Source: CAD feature listing. Evaluate the final solid. Frame: model axes, mm. Face numbers are marked on the shaded views. Round coordinates to 2 decimals unless told otherwise and drop trailing zeros. Order: outer loops, then holes, each group sorted by start corner. A loop starts at its lowest first (then second) coordinate and runs counter-clockwise, first axis right, second up. Notation, with made-up numbers: (6, 38) -> (46, 38) arc R28 cw to (46, 62) -> close; hole circle Ø1 at (40, 88). An arc over 180 degrees is marked (long way). Write item = value, one per line. Start each with the question number.
(1) Cut plane C-C on z = 12. Return the cut outline in (x, y) (3 decimals), then the cut area to 3 significant figures.
(2) Ray query, line 1 (Y direction, x = 11.71, z = 0.6); line 2 (X direction, y = 2.75, z = 1); line 3 (Y direction, x = 11.71, z = 5.75). Return the intervals inside material, ascending.
(3) Contact query for a flat-ended pin moving along its axis: pin 1 Ø2 at (x, y) = (8.5, 1) entering from +Z. Output: stop coordinate, or through.
(4) Cut plane A-A on x = 27.29. Return the cut outline in (y, z).
(5) Cut plane B-B on z = 3. Return the cut outline in (x, y) (3 decimals), then the cut area to 3 significant figures.
(6) Draft query along Y for the marked faces 1, 2, 3 and 4. Return one class per face: released by +Y, released by -Y, zero draft, split by the parting line, or undercut.
(7) Cut plane D-D on y = 3. Give the number of separate pieces and of enclosed holes in the cut face, then the cut area to 3 significant figures.
from build123d import *

# Parameters (mm, degrees)
SKETCH1_W                = 39
SKETCH1_H                = 7.38
BOSS_EXTRUDE1_DEPTH      = 7.76
SKETCH2_R                = 2.4
CUT_EXTRUDE1_DEPTH       = 7.76
CUT_EXTRUDE2_OUTLINE_R   = 3.1
CUT_EXTRUDE2_OUTLINE_R_2 = 2.4
CUT_EXTRUDE2_DEPTH       = 0.8
CUT_EXTRUDE3_START       = 6.96
CUT_EXTRUDE3_OUTLINE_R   = 3.1
CUT_EXTRUDE3_OUTLINE_R_2 = 2.4
CUT_EXTRUDE3_DEPTH       = 0.8
LPATTERN3_COUNT          = 3
LPATTERN3_PITCH          = 7.79
LPATTERN6_COUNT          = 3
LPATTERN6_PITCH          = 7.79
FILLET1_R                = 3.69
FILLET2_R                = 3.69
FILLET3_R                = 3.69
FILLET4_R                = 3.69
SKETCH3_R                = 3.1
BOSS_EXTRUDE2_DEPTH      = 7.76
BOSS_EXTRUDE3_START      = -7.76
SKETCH4_R                = 3.1
BOSS_EXTRUDE3_DEPTH      = 7.76
SKETCH11_R               = 1.555
BOSS_EXTRUDE7_DEPTH      = 8
SKETCH12_R               = 1.555
BOSS_EXTRUDE8_DEPTH      = 8
SKETCH14_R               = 1.555
BOSS_EXTRUDE9_DEPTH      = 8


# Read off the part's stored shape, not the designer's step: Cut-Extrude2, Cut-Extrude3
with BuildPart() as part:
    # Sketch1 → Boss-Extrude1 (new body)
    with BuildSketch(Plane.XY):
        with Locations((19.5, 3.69)):
            Rectangle(SKETCH1_W, SKETCH1_H)
    extrude(amount=BOSS_EXTRUDE1_DEPTH)

    # Sketch2 → Cut-Extrude1 (cut)
    with BuildSketch(Plane.XY.offset(7.76)):
        with Locations((19.5, 3.69)):
            Circle(SKETCH2_R)
    cut_extrude1 = extrude(amount=-CUT_EXTRUDE1_DEPTH, mode=Mode.SUBTRACT)

    # Cut-Extrude2 outline → Cut-Extrude2 (cut)
    with BuildSketch(Plane.XY):
        with Locations((19.5, 3.69)):
            Circle(CUT_EXTRUDE2_OUTLINE_R)
        with Locations((19.5, 3.69)):
            Circle(CUT_EXTRUDE2_OUTLINE_R_2, mode=Mode.SUBTRACT)
    cut_extrude2 = extrude(amount=CUT_EXTRUDE2_DEPTH, mode=Mode.SUBTRACT)

    # Cut-Extrude3 outline → Cut-Extrude3 (cut)
    with BuildSketch(Plane.XY.offset(CUT_EXTRUDE3_START)):
        with Locations((19.5, 3.69)):
            Circle(CUT_EXTRUDE3_OUTLINE_R)
        with Locations((19.5, 3.69)):
            Circle(CUT_EXTRUDE3_OUTLINE_R_2, mode=Mode.SUBTRACT)
    cut_extrude3 = extrude(amount=CUT_EXTRUDE3_DEPTH, mode=Mode.SUBTRACT)

    # LPattern3: Cut-Extrude1, Cut-Extrude2, Cut-Extrude3 ×3
    with Locations(*[(-i * LPATTERN3_PITCH, 0, 0) for i in range(1, LPATTERN3_COUNT)]):
        add(cut_extrude1, mode=Mode.SUBTRACT)
        add(cut_extrude2, mode=Mode.SUBTRACT)
        add(cut_extrude3, mode=Mode.SUBTRACT)

    # LPattern6: Cut-Extrude1, Cut-Extrude2, Cut-Extrude3 ×3
    with Locations(*[(i * LPATTERN6_PITCH, 0, 0) for i in range(1, LPATTERN6_COUNT)]):
        add(cut_extrude1, mode=Mode.SUBTRACT)
        add(cut_extrude2, mode=Mode.SUBTRACT)
        add(cut_extrude3, mode=Mode.SUBTRACT)

    # Fillet1
    fillet1_edges = [part.edges().sort_by_distance(p)[0] for p in [
        (0, 7.38, 3.88),
    ]]
    fillet(fillet1_edges, radius=FILLET1_R)

    # Fillet2
    fillet2_edges = [part.edges().sort_by_distance(p)[0] for p in [
        (0, 0, 3.88),
    ]]
    fillet(fillet2_edges, radius=FILLET2_R - 0.0001)  # a hair under: the kernel refuses the full size

    # Fillet3
    fillet3_edges = [part.edges().sort_by_distance(p)[0] for p in [
        (39, 7.38, 3.88),
    ]]
    fillet(fillet3_edges, radius=FILLET3_R)

    # Fillet4
    fillet4_edges = [part.edges().sort_by_distance(p)[0] for p in [
        (39, 0, 3.88),
    ]]
    fillet(fillet4_edges, radius=FILLET4_R - 0.0001)  # a hair under: the kernel refuses the full size

    # Sketch3 → Boss-Extrude2 (add)
    with BuildSketch(Plane(origin=(0, 0, 0), x_dir=(-1, 0, 0), z_dir=(0, 0, -1))):
        with Locations((-35.08, 3.69)):
            Circle(SKETCH3_R)
    extrude(amount=-BOSS_EXTRUDE2_DEPTH)

    # Sketch4 → Boss-Extrude3 (add)
    with BuildSketch(Plane.XY.offset(7.76).offset(BOSS_EXTRUDE3_START)):
        with Locations((3.92, 3.69)):
            Circle(SKETCH4_R)
    extrude(amount=BOSS_EXTRUDE3_DEPTH)

    # Sketch11 → Boss-Extrude7 (add)
    with BuildSketch(Plane.XY.offset(7.76)):
        with Locations(Location((0.085, 3.69, 0), (0, 0, 279.228133411))):
            Circle(SKETCH11_R)
        with Locations(Location((38.915, 3.69, 0), (0, 0, 99.228133411))):
            Circle(SKETCH11_R)
    extrude(amount=BOSS_EXTRUDE7_DEPTH)

    # Sketch12 → Boss-Extrude8 (add)
    with BuildSketch(Plane(origin=(0, 0, 0), x_dir=(-1, 0, 0), z_dir=(0, 0, -1))):
        with Locations(Location((-38.915, 3.69, 0), (0, 0, 80.771866589))):
            Circle(SKETCH12_R)
    extrude(amount=-BOSS_EXTRUDE8_DEPTH)

    # Sketch14 → Boss-Extrude9 (add)
    with BuildSketch(Plane(origin=(0, 0, 0), x_dir=(-1, 0, 0), z_dir=(0, 0, -1))):
        with Locations(Location((-0.085, 3.69, 0), (0, 0, 99.228133411))):
            Circle(SKETCH14_R)
    extrude(amount=-BOSS_EXTRUDE9_DEPTH)


solid = part.part
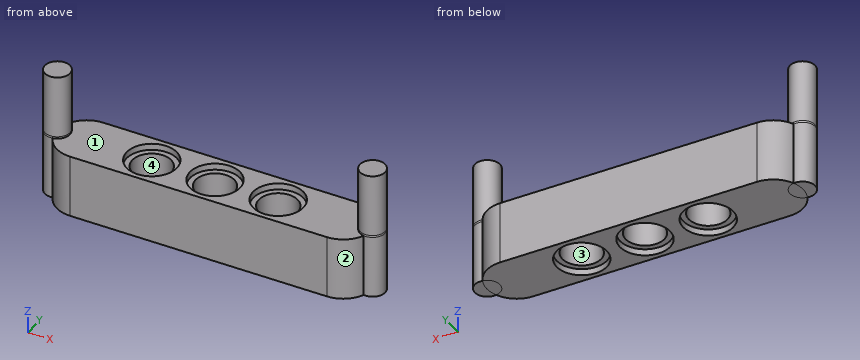
Evaluation:
q1.outline = circle Ø3.11 at (0.085, 3.69); circle Ø3.11 at (38.915, 3.69)
q1.area = 15.2 mm^2
q2.line_1 = 0 to 0.59, 6.79 to 7.38
q2.line_2 = -1.15 to 9.5, 13.92 to 17.29, 21.71 to 25.08, 29.5 to 40.15
q2.line_3 = 0 to 1.29, 6.09 to 7.38
q3.pin_1 = 7.76
q4.outline = (0, 0) -> (0.59, 0) -> (0.59, 0.8) -> (1.29, 0.8) -> (1.29, 6.96) -> (0.59, 6.96) -> (0.59, 7.76) -> (0, 7.76) -> close; (6.09, 0.8) -> (6.79, 0.8) -> (6.79, 0) -> (7.38, 0) -> (7.38, 7.76) -> (6.79, 7.76) -> (6.79, 6.96) -> (6.09, 6.96) -> close
q5.outline = (0.334, 2.155) arc R3.69 ccw to (3.69, 0) -> (35.31, 0) arc R3.69 ccw to (38.666, 2.155) arc R1.555 ccw (long way) to (38.666, 5.225) arc R3.69 ccw to (35.31, 7.38) -> (3.69, 7.38) arc R3.69 ccw to (0.334, 5.225) arc R1.555 ccw (long way) to start; hole circle Ø4.8 at (11.71, 3.69); hole circle Ø4.8 at (19.5, 3.69); hole circle Ø4.8 at (27.29, 3.69)
q5.area = 230 mm^2
q6.face_1 = zero draft
q6.face_2 = released by -Y
q6.face_3 = undercut
q6.face_4 = undercut
q7.separate_pieces = 4
q7.enclosed_holes = 0
q7.area = 254 mm^2
